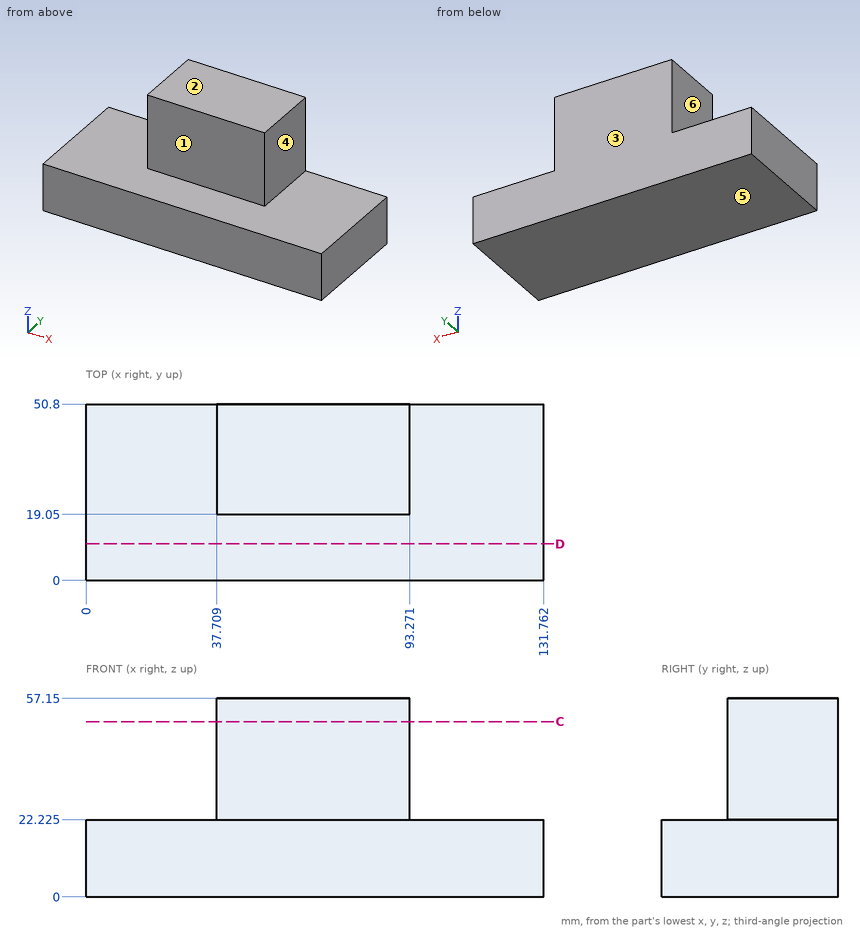
Geometry check sheet. Reference: drawing and pictorial views, mm from the part's lowest x, y, z. A direction names the side the tool comes from. Coordinates: 2 decimals unless noted, no trailing zeros. Order: outer loops, then holes, each group sorted by start corner. A loop starts at its lowest first (then second) coordinate and runs counter-clockwise, first axis right, second up.
Item 1: Access from +Z, -Z, +X, -X, +Y, -Y to the whole of each face (thin tool, end or side, straight path). Record for the marked faces 4, 5 and 6.
Filled in:
face 4: +Z, +X, +Y, -Y
face 5: -Z, +X, -X, +Y, -Y
face 6: +Z, -X, +Y, -Y
Item 2: Section check D-D, the plane y = 10.5. Enter the section's corners in (x, z) (1 decimal), then the cut area to 3 significant figures.
Filled in:
outline: (0, 0) - (131.8, 0) - (131.8, 22.2) - (0, 22.2) - close
area: 2,930 mm2
Item 3: Release check for a two-part mould opening along Y. For the marked faces 1, 2 and 3 record: +Y half, -Y half, draft (parallel to the pull), parting line (faces both ways), or undercut.
Filled in:
face 1: -Y half
face 2: draft
face 3: +Y half
Item 4: Material ranges on L1, parallel to Z at x = 20, y = 39 (1 decimal); L2, parallel to Y at x = 70, z = 37; L3, parallel to X at y = 22, z = 49, recorded low to high.
Filled in:
L1: z = 0 to 22.2
L2: y = 19.05 to 50.8
L3: x = 37.71 to 93.27
Item 5: Section check C-C, the plane z = 50.5. Enter the section's corners in (x, y).
Filled in:
outline: (37.71, 19.05) - (93.27, 19.05) - (93.27, 50.8) - (37.71, 50.8) - close
Item 6: Depth check by flat-ended pin: pin 1 (5 mm diameter, centred on x = 105, y = 41.5, fed in from -Z); pin 2 (2 mm diameter, centred on y = 29, z = 24, fed in from -X); pin 3 (6 mm diameter, centred on x = 101, y = 36.5, fed in from +Z) (1 decimal); pin 4 (5 mm diameter, centred on y = 39, z = 50, fed in from +X). Enter the tip coordinate at first touch or a pass-through.
Filled in:
pin 1: stops at z = 0
pin 2: stops at x = 37.71
pin 3: stops at z = 22.2
pin 4: stops at x = 93.27
